```python
from build123d import *

# Parameters (mm, degrees)
SKETCH2_R      = 5
EXTRUDE1_DEPTH = 20
SKETCH3_R      = 1.5
EXTRUDE2_DEPTH = 15


with BuildPart() as part:
    # Sketch1 → Revolve1 (revolve)
    with BuildSketch(Plane.XY):
        Polygon((0, 86.10058483), (14, 86.10058483), (14, 81.10058483), (23.5, 55.889277686), (25.5, 42.889277686), (25.5, 36.10058483), (27.5, 36.10058483), (27.5, 18.10058483), (25.5, 18.10058483), (25.5, -7.110722314), (23.5, -23.39941517), (23.5, -63.39941517), (12, -74.89941517), (9, -74.89941517), (9, -86.89941517), (5, -86.89941517), (5, -103.89941517), (0, -103.89941517), align=None)
    revolve(axis=Axis((0, 86.10058483, 0), (0, -1, 0)))

    # Sketch2 → Extrude1 (add)
    with BuildSketch(Plane(origin=(0, 86.10058483, 0), x_dir=(1, 0, 0), z_dir=(0, 1, 0))):
        Circle(SKETCH2_R)
    extrude(amount=EXTRUDE1_DEPTH)

    # Sketch3 → Extrude2 (add)
    with BuildSketch(Plane.XZ.offset(103.89941517)):
        Circle(SKETCH3_R)
    extrude(amount=EXTRUDE2_DEPTH)


solid = part.part
```
Geometry: final body of the model. Coordinates: model frame, mm. A direction names the side the tool comes from. Round coordinates to 2 decimals unless told otherwise and drop trailing zeros. Order: outer loops, then holes, each group sorted by start corner. A loop starts at its lowest first (then second) coordinate and runs counter-clockwise, first axis right, second up. Notation, with made-up numbers: (-14.75, 63) -> (-1.75, 63) arc R27 ccw to (-1.75, 84) -> close; hole circle Ø4 at (5.5, 32). An arc over 180 degrees is marked (long way). Use one line per item in the form item = value. Start each with the question number.
1. Cut plane A-A (y = -99). Return the cut outline in (x, z).
2. Cut plane B-B (y = -2). Return the cut outline in (x, z), then the cut area to 3 significant figures.
3. Line query: probe 1 along Y at (x, z) = (2.5, 10); probe 2 along Y at (x, z) = (-4.5, -7); probe 3 along X at (y, z) = (51, -0.5). Output: solid intervals per line, ascending.
4. Pin query (flat end, axial travel): pin 1 Ø1 at (y, z) = (8.5, 21.5) entering from -X; pin 2 Ø12 at (x, y) = (1, 9.5) entering from -Z; pin 3 Ø6 at (y, z) = (-86.5, 10.5) entering from +X. Return the tip coordinate at first contact, or that it passes through.
5. Reachability of faces 1 (the face through (2, -74.899, 9)), 2 (the face through (-1.08, 95.96, 4.88)), 3 (the face through (-5.961, 26.975, -26.846)) from +Z, -Z, +X, -X, +Y, -Y: full face, straight path, thin tool, end or side. Return the list, or none.
Solution:
q1.outline = circle Ø10 at (0, 0)
q2.outline = circle Ø51 at (0, 0)
q2.area = 2,040 mm^2
q3.probe_1 = -74.9 to 86.1
q3.probe_2 = -86.9 to 86.1
q3.probe_3 = -24.25 to 24.25
q4.pin_1 = -14.47
q4.pin_2 = -25.5
q4.pin_3 = 4.97
q5.face_1 = -Y
q5.face_2 = +Y
q5.face_3 = +Y, -Y
